```python
from build123d import *

# Parameters (mm, degrees)
HOUSING_2_DEPTH          = 44.45
SKETCH2_R                = 36.6649
IMPELLER_CUT_DEPTH       = 22.4028
SKETCH4_R                = 4.826
INLET_CUT_DEPTH          = 19.8628
SKETCH6_R                = 3.175
FASTENER_BORE_DEPTH      = 116.84
FASTENER_PATTERN_COUNT   = 8
SKETCH7_R                = 100.114274451
SKETCH7_R_2              = 19.05
MASS_REDUCTION_CUT_DEPTH = 10.414
SKETCH11_R               = 19.05
SKETCH11_R_2             = 4.826
BOSS_EXTRUDE1_DEPTH      = 6.35
SKETCH14_R               = 2.38125
CUT_EXTRUDE3_DEPTH       = 99.06
SKETCH15_R               = 9.525
CUT_EXTRUDE4_DEPTH       = 25.4
BOSS_EXTRUDE2_START      = 12.7
SKETCH16_R               = 9.525
SKETCH16_R_2             = 6.35
BOSS_EXTRUDE2_DEPTH      = 12.7
SKETCH18_W               = 6.604
SKETCH18_H               = 47.625
BOSS_EXTRUDE3_DEPTH      = 19.05
SKETCH19_R               = 2.5781
CUT_EXTRUDE5_DEPTH       = 17.78
CIRPATTERN2_COUNT        = 4
FILLET9_R                = 6.35
SKETCH22_R               = 8.9281
CUT_EXTRUDE8_DEPTH       = 17.78
CHAMFER1_SIZE            = 3.175


with BuildPart() as part:
    # Sketch1 → Housing 2 (new body)
    with BuildSketch(Plane(origin=(0, 0, 0), x_dir=(0, 0, -1), z_dir=(1, 0, 0))):
        with BuildLine():
            Line((-60.96, 0), (-60.96, 60.96))
            Line((-60.96, 60.96), (0, 60.96))
            ThreePointArc((0, 60.96), (31.907091375, 51.942844743), (54.374839025, 27.559))
            Line((54.374839025, 27.559), (60.96, 27.559))
            Line((60.96, 27.559), (60.96, -27.559))
            Line((60.96, -27.559), (54.374839025, -27.559))
            ThreePointArc((54.374839025, -27.559), (43.093739421, -43.116716279), (27.530012063, -54.389521379))
            Line((27.530012063, -54.389521379), (27.530012063, -60.96))
            Line((27.530012063, -60.96), (-27.530012063, -60.96))
            Line((-27.530012063, -60.96), (-27.530012063, -54.389521379))
            ThreePointArc((-27.530012063, -54.389521379), (-51.934339003, -31.920934077), (-60.96, 0))
        make_face()
    extrude(amount=HOUSING_2_DEPTH)

    # Sketch2 → Impeller Cut (cut)
    with BuildSketch(Plane.ZY):
        Circle(SKETCH2_R)
    extrude(amount=-IMPELLER_CUT_DEPTH, mode=Mode.SUBTRACT)

    # Sketch3 → Impeller Angle Cut (revolve, cut)
    with BuildSketch(Plane.XY, mode=Mode.PRIVATE) as impeller_angle_cut_sk:
        Polygon((28.08333914, 9.28793198), (22.4028, 36.6649), (22.225, 0), (28.08333914, 0), align=None)
    revolve(impeller_angle_cut_sk.sketch.rotate(Axis((22.225, 0, 0), (1, 0, 0)), 180), axis=Axis((22.225, 0, 0), (1, 0, 0)), mode=Mode.SUBTRACT)

    # Sketch4 → Inlet Cut (cut)
    with BuildSketch(Plane.ZY.offset(-28.08333914)):
        Circle(SKETCH4_R)
    extrude(amount=-INLET_CUT_DEPTH, mode=Mode.SUBTRACT)

    # Sketch6 → Fastener Bore (cut)
    with BuildSketch(Plane(origin=(44.45, 0, 0), x_dir=(0, 0, -1), z_dir=(1, 0, 0))):
        with Locations((50.8, 0)):
            Circle(SKETCH6_R)
    fastener_bore = extrude(amount=-FASTENER_BORE_DEPTH, mode=Mode.SUBTRACT)

    # Fastener Pattern: Fastener Bore ×8 about axis, 1 skipped
    fastener_pattern_axis = Axis((0, 0, 0), (-1, 0, 0))
    add([fastener_bore.rotate(fastener_pattern_axis, i * 360 / FASTENER_PATTERN_COUNT) for i in range(1, FASTENER_PATTERN_COUNT) if i not in (5,)], mode=Mode.SUBTRACT)

    # Sketch7 → Mass Reduction Cut (cut)
    with BuildSketch(Plane(origin=(44.45, 0, 0), x_dir=(0, 0, -1), z_dir=(1, 0, 0))):
        Circle(SKETCH7_R)
        Circle(SKETCH7_R_2, mode=Mode.SUBTRACT)
    extrude(amount=-MASS_REDUCTION_CUT_DEPTH, mode=Mode.SUBTRACT)

    # Sketch11 → Boss-Extrude1 (add)
    with BuildSketch(Plane(origin=(44.45, 0, 0), x_dir=(0, 0, -1), z_dir=(1, 0, 0))):
        Circle(SKETCH11_R)
        with Locations(Location((0, 0, 0), (0, 0, 180))):
            Circle(SKETCH11_R_2, mode=Mode.SUBTRACT)
    extrude(amount=BOSS_EXTRUDE1_DEPTH)

    # Sketch14 → Cut-Extrude3 (cut)
    with BuildSketch(Plane.XY):
        with Locations(Location((18.415, 30.734, 0), (0, 0, 180))):
            Circle(SKETCH14_R)
    extrude(amount=CUT_EXTRUDE3_DEPTH, mode=Mode.SUBTRACT)

    # Sketch15 → Cut-Extrude4 (cut)
    with BuildSketch(Plane.XY.offset(60.96)):
        with Locations((18.415, 30.734)):
            Circle(SKETCH15_R)
    extrude(amount=-CUT_EXTRUDE4_DEPTH, mode=Mode.SUBTRACT)

    # Sketch16 → Boss-Extrude2 (add)
    with BuildSketch(Plane.XY.offset(35.56).offset(BOSS_EXTRUDE2_START)):
        with Locations((18.415, 30.734)):
            Circle(SKETCH16_R)
        with Locations(Location((18.415, 30.734, 0), (0, 0, 180))):
            Circle(SKETCH16_R_2, mode=Mode.SUBTRACT)
    extrude(amount=-BOSS_EXTRUDE2_DEPTH)

    # Sketch18 → Boss-Extrude3 (add)
    with BuildSketch(Plane.XY.offset(60.96)):
        with Locations((37.338, 37.1475)):
            Rectangle(SKETCH18_W, SKETCH18_H)
    extrude(amount=-BOSS_EXTRUDE3_DEPTH)

    # Sketch19 → Cut-Extrude5 (cut)
    with BuildSketch(Plane.XY.offset(60.96)):
        with Locations((30.987358569, 18.161641431)):
            Circle(SKETCH19_R)
    cut_extrude5 = extrude(amount=-CUT_EXTRUDE5_DEPTH, mode=Mode.SUBTRACT)

    # CirPattern2: Cut-Extrude5 ×4 about axis
    cirpattern2_axis = Axis((18.415, 30.734, 0), (0, 0, 1))
    for i in range(1, CIRPATTERN2_COUNT):
        add(cut_extrude5.rotate(cirpattern2_axis, i * 360 / CIRPATTERN2_COUNT), mode=Mode.SUBTRACT)

    # Fillet9
    fillet9_edges = [part.edges().sort_by_distance(p)[0] for p in [
        (17.018, 27.559, -54.374839025),
        (17.018, -27.559, -54.374839025),
        (17.018, -54.389521379, -27.530012063),
        (17.018, -54.389521379, 27.530012063),
    ]]
    fillet(fillet9_edges, radius=FILLET9_R)

    # Sketch22 → Cut-Extrude8 (cut)
    with BuildSketch(Plane(origin=(50.8, 0, 0), x_dir=(0, 0, -1), z_dir=(1, 0, 0))):
        Circle(SKETCH22_R)
    extrude(amount=-CUT_EXTRUDE8_DEPTH, mode=Mode.SUBTRACT)

    # Chamfer1
    chamfer1_edges = [part.edges().sort_by_distance(p)[0] for p in [
        (50.8, 0, 19.05),
    ]]
    chamfer(chamfer1_edges, length=CHAMFER1_SIZE)


solid = part.part
```
CAD build for the part. Positions are in the model's coordinates, mm. A direction names the side the tool comes from. Round coordinates to 2 decimals unless told otherwise and drop trailing zeros. Write each loop counter-clockwise with the first axis right and the second up, starting at its lowest first coordinate (ties: lowest second). Pieces come first, ordered by that corner, then holes.
Item 1: Tool access for faces 5 (the flat face through (37, 13.335, 52)), 6 (the cylindrical face through (11.045, -35.793, -7.948)), 7 (the flat face through (6, 18, 43.18)), 8 (the cylindrical face through (17.256, 28.426, -54.942)), 9 (the flat face through (33.02, -4, -4)): list every direction of +Z, -Z, +X, -X, +Y, -Y with a clear straight run to the whole face (end or side of a thin tool).
Filled in:
face 5: +Z, +X, -Y
face 6: -X
face 7: +Z
face 8: -Z, +X, -X, +Y
face 9: +X
Item 2: Drop flat-ended pins along their axis: pin 1 Ø3 at (y, z) = (-18.5, 8) entering from +X; pin 2 Ø3 at (x, y) = (30.99, 43.31) entering from -Z; pin 3 Ø22 at (x, y) = (18.415, 30.734) entering from -Z; pin 4 Ø1.5 at (x, y) = (30, 44.5) entering from +Z. Give the stop position or say it passes through.
Filled in:
pin 1: stops at x = 48.02
pin 2: stops at z = -44.36
pin 3: stops at z = -60.96
pin 4: stops at z = 43.18
Item 3: Mould opens along X. For faces 1 (the flat face through (20, 60.96, 31)), 2 (the cylindrical face through (17.18, 40.18, 54.7)), 3 (the flat face through (6, 43, 43.18)), 4 (the flat face through (0, 28, 26)) say: released by +X, released by -X, zero draft, split by the parting line, or undercut.
Filled in:
face 1: zero draft
face 2: undercut
face 3: undercut
face 4: released by -X
Item 4: Band-saw the part on B-B on x = 45. Write the cut outline in (y, z), then the cut area to 3 significant figures.
Filled in:
outline: circle Ø38.1 at (0, 0); hole circle Ø17.86 at (0, 0)
area: 890 mm2
Item 5: Band-saw the part on C-C on y = -50.8. Write the cut outline in (x, z) (3 decimals).
Filled in:
outline: (0, -33.697) - (34.036, -33.697) - (34.036, -3.175) - (0, -3.175) - close; (0, 3.175) - (34.036, 3.175) - (34.036, 33.697) - (0, 33.697) - close
Item 6: Band-saw the part on A-A on z = 50.8. Write the cut outline in (x, y) (3 decimals).
Filled in:
outline: (0, -33.697) - (34.036, -33.697) - (34.036, -3.175) - (0, -3.175) - close; (0, 3.175) - (34.036, 3.175) - (34.036, 13.335) - (40.64, 13.335) - (40.64, 60.96) - (0, 60.96) - close; hole circle Ø5.156 at (5.843, 18.162); hole circle Ø5.156 at (5.843, 43.306); hole circle Ø19.05 at (18.415, 30.734); hole circle Ø5.156 at (30.987, 18.162); hole circle Ø5.156 at (30.987, 43.306)
Item 7: Drill centre lines: L1, parallel to Z at x = 9, y = -38.5; L2, parallel to Y at x = 15, z = 50; L3, parallel to X at y = -33, z = 44. Where is each one in solid material? Low to high.
Filled in:
L1: z = -47.26 to -37.77, -34.07 to 34.07, 37.77 to 47.26
L2: y = -34.87 to -3.07, 3.07 to 21.84, 39.63 to 60.96
L3: x = 0 to 34.04
